Can you work these out from the drawing? Everything is in mm from the part's minimum corner. Give positions to 0.01 mm unless a question says otherwise; leave off trailing zeros. Write each loop counter-clockwise with the first axis right and the second up, starting at its lowest first coordinate (ties: lowest second). Pieces come first, ordered by that corner, then holes. Notation, with made-up numbers: (27, -26.75) - (54, -26.75) arc R38 ccw to (54, 12.25) - close; hole circle Ø2 at (86.5, 86). An arc over 180 degrees is marked (long way). Use a Markdown table: item, result.
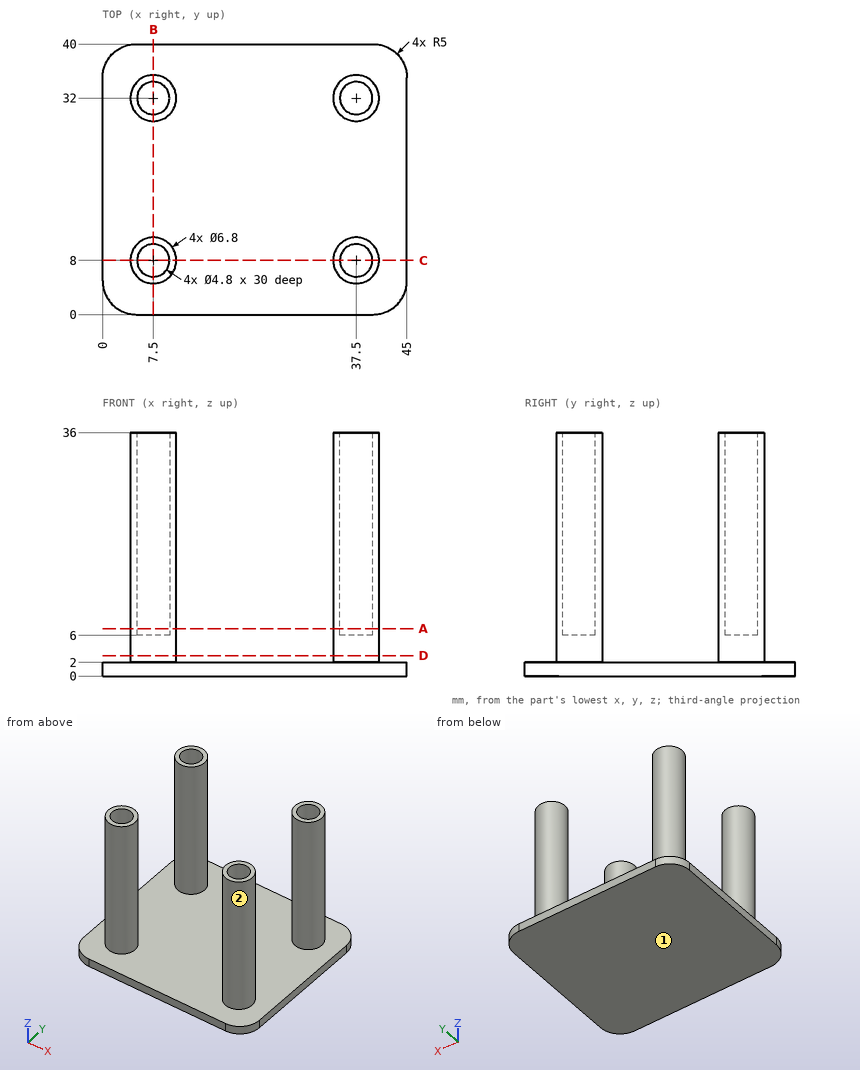
Item 1: I need wall thicknesses on line 1 along Y through (x, z) = (7.5, 12.75); line 2 along Y through (x, z) = (7, 23); line 3 along X through (y, z) = (8.5, 12). Which ranges of each line are inside material? Lowest first, please. Write a range as [from, to].
Values:
| item | result |
|---|---|
| line 1 | y = [4.6, 5.6], [10.4, 11.4], [28.6, 29.6], [34.4, 35.4] |
| line 2 | y = [4.64, 5.65], [10.35, 11.36], [28.64, 29.65], [34.35, 35.36] |
| line 3 | x = [4.14, 5.15], [9.85, 10.86], [34.14, 35.15], [39.85, 40.86] |
Item 2: Will these pins go through, and if not, where does the flat tip stop? pin 1 Ø1.4 at (x, y) = (37, 7.5) entering from +Z; pin 2 Ø10 at (y, z) = (26.5, 15.5) entering from -X; pin 3 Ø12 at (y, z) = (24.5, 24) entering from -X; pin 4 Ø4 at (x, y) = (7.5, 32) entering from -Z.
Values:
| item | result |
|---|---|
| pin 1 | stops at z = 6 |
| pin 2 | stops at x = 4.14 |
| pin 3 | stops at x = 4.45 |
| pin 4 | stops at z = 0 |
Item 3: If we section it at C-C, the plane y = 8: Write out the boundary of the cut face in (x, z).
Values:
| item | result |
|---|---|
| outline | (0, 0) - (45, 0) - (45, 2) - (40.9, 2) - (40.9, 36) - (39.9, 36) - (39.9, 6) - (35.1, 6) - (35.1, 36) - (34.1, 36) - (34.1, 2) - (10.9, 2) - (10.9, 36) - (9.9, 36) - (9.9, 6) - (5.1, 6) - (5.1, 36) - (4.1, 36) - (4.1, 2) - (0, 2) - close |
Item 4: Thinking about a two-plate mould opening in Y: for the marked faces 1 and 2, which applies, +Y half, -Y half, draft (parallel to the pull), parting line (faces both ways), or undercut?
Values:
| item | result |
|---|---|
| face 1 | draft |
| face 2 | undercut |
Item 5: If we section it at D-D, the plane z = 3: Write out the boundary of the cut face in (x, y).
Values:
| item | result |
|---|---|
| outline | circle Ø6.8 at (7.5, 8); circle Ø6.8 at (7.5, 32); circle Ø6.8 at (37.5, 8); circle Ø6.8 at (37.5, 32) |
Item 6: If we section it at A-A, the plane z = 7: Write out the boundary of the cut face in (x, y), plus the area to 3 significant figures.
Values:
| item | result |
|---|---|
| outline | circle Ø6.8 at (7.5, 8); circle Ø6.8 at (7.5, 32); circle Ø6.8 at (37.5, 8); circle Ø6.8 at (37.5, 32); hole circle Ø4.8 at (7.5, 8); hole circle Ø4.8 at (7.5, 32); hole circle Ø4.8 at (37.5, 8); hole circle Ø4.8 at (37.5, 32) |
| area | 72.9 mm2 |
Item 7: If we section it at B-B, the plane x = 7.5: Write out the boundary of the cut face in (y, z).
Values:
| item | result |
|---|---|
| outline | (0, 0) - (40, 0) - (40, 2) - (35.4, 2) - (35.4, 36) - (34.4, 36) - (34.4, 6) - (29.6, 6) - (29.6, 36) - (28.6, 36) - (28.6, 2) - (11.4, 2) - (11.4, 36) - (10.4, 36) - (10.4, 6) - (5.6, 6) - (5.6, 36) - (4.6, 36) - (4.6, 2) - (0, 2) - close |
